Source: CAD feature listing. Evaluate the final solid. Frame: model axes, mm. Round coordinates to 2 decimals unless told otherwise and drop trailing zeros. Loops run counter-clockwise (first coordinate to the right, second up) from the corner with the lowest first, then second, coordinate; pieces in that order, holes last. Notation, with made-up numbers: (-20.75, -35) - (29.25, -35) arc R36 ccw to (29.25, 3) - close; hole circle Ø10 at (87.5, 55.25). An arc over 180 degrees is marked (long way). One line per question, with ' | ' between items. Start each with the question number.
1. Ray query, line 1 (Z direction, x = 267, y = 8.5); line 2 (Z direction, x = -224, y = 4); line 3 (Z direction, x = -98, y = 8). Return the intervals inside material, ascending.
2. Cut plane A-A (y = 7.75). Return loops of the section in (x, z) (3 decimals), then the cut area to 3 significant figures.
3. Cut plane B-B (z = -375.5). Return loops of the section in (x, y), then the cut area to 3 significant figures.
4. Cut plane C-C (x = -111). Return loops of the section in (y, z), then the cut area to 3 significant figures.
5. Pin query (flat end, axial travel): pin 1 (2 mm diameter, centred on x = 553.5, y = 5, fed in from +Z); pin 2 (2 mm diameter, centred on y = 5.5, z = -61.5, fed in from +X); pin 3 (2.5 mm diameter, centred on y = 6.5, z = -517.5, fed in from -X). Return the tip coordinate at first contact, or that it passes through.
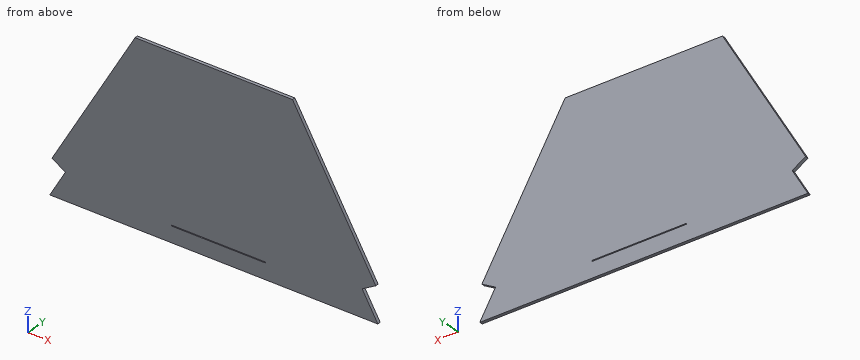
```python
from build123d import *

# Parameters (mm, degrees)
BOSS_EXTRUDE1_DEPTH = 10
SKETCH2_W           = 300
SKETCH2_H           = 3
CUT_EXTRUDE1_DEPTH  = 959.755029562


with BuildPart() as part:
    # Sketch1 → Boss-Extrude1 (new body)
    with BuildSketch(Plane(origin=(0, 0, 0), x_dir=(1, 0, 0), z_dir=(0, 1, 0))):
        Polygon((-271.133729811, 569.617395678), (771.133729811, 569.617395678), (721.133729811, 483.014855299), (764.435, 458.014855299), (500, 0), (0, 0), (-264.435, 458.014855299), (-221.133729811, 483.014855299), align=None)
    extrude(amount=BOSS_EXTRUDE1_DEPTH)

    # Sketch2 → Cut-Extrude1 (cut, through all)
    with BuildSketch(Plane.XZ):
        with Locations((264.88, -518.12)):
            Rectangle(SKETCH2_W, SKETCH2_H)
    extrude(amount=-CUT_EXTRUDE1_DEPTH, mode=Mode.SUBTRACT)


solid = part.part
```
Answers follow:
1) line 1: z = -569.62 to -519.62, -516.62 to 0 | line 2: z = -569.62 to -487.98, -481.36 to -387.98 | line 3: z = -569.62 to -169.74
2) outline: (-271.134, -569.617) - (771.134, -569.617) - (721.134, -483.015) - (764.435, -458.015) - (500, 0) - (0, 0) - (-264.435, -458.015) - (-221.134, -483.015) - close; hole (114.88, -519.62) - (414.88, -519.62) - (414.88, -516.62) - (114.88, -516.62) - close | area: 460,000 mm2
3) outline: (-216.8, 0) - (716.8, 0) - (716.8, 10) - (-216.8, 10) - close | area: 9,340 mm2
4) outline: (0, -569.62) - (10, -569.62) - (10, -192.26) - (0, -192.26) - close | area: 3,770 mm2
5) pin 1: stops at z = -90.93 | pin 2: stops at x = 536.08 | pin 3: stops at x = -241.77
